from build123d import *

# Parameters (mm, degrees)
PAD_DEPTH   = 3.175
SKETCH001_R = 1.7
HOLE_DEPTH  = 3.176


with BuildPart() as part:
    # Sketch → Pad (new body)
    with BuildSketch(Plane.XY):
        with BuildLine():
            ThreePointArc((0, 3), (-3, 0), (0, -3))
            Line((0, -3), (35, -3))
            ThreePointArc((35, -3), (38, 0), (35, 3))
            Line((0, 3), (35, 3))
        make_face()
    extrude(amount=PAD_DEPTH)

    # Sketch001 (on Face6 of Pad) → Hole (cut, through all)
    with BuildSketch(Plane.XY.offset(3.175)):
        Circle(SKETCH001_R)
        with Locations((35, 0)):
            Circle(SKETCH001_R)
    extrude(amount=-HOLE_DEPTH, mode=Mode.SUBTRACT)


solid = part.part
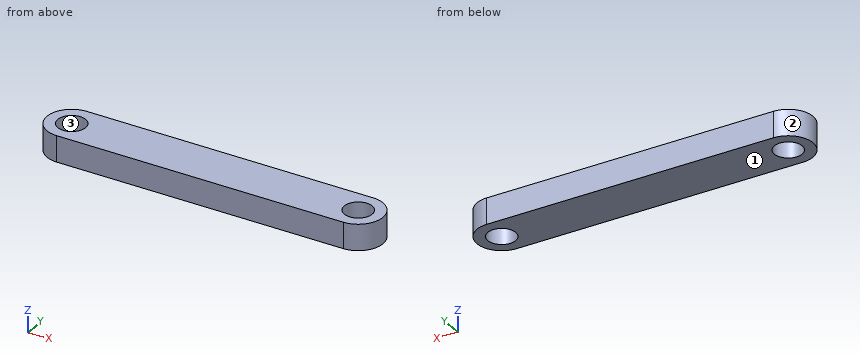
The listing builds one solid part. Answer for the finished solid, in the listing's coordinates (mm). Face numbers are marked on the shaded views. Coordinates: 2 decimals unless noted, no trailing zeros. Write each loop counter-clockwise with the first axis right and the second up, starting at its lowest first coordinate (ties: lowest second). Pieces come first, ordered by that corner, then holes. Notation, with made-up numbers: M 10.5,69.25 L 48.5,69.25 A25 cw 48.5,96.25 Z; hole C -12,-23 d1. An arc over 180 degrees is marked long. Write each question's results on one line, items separated by ' | '.
Item 1: For a pull along X with two mould halves and no side action, classify the marked faces 1, 2 and 3 as released by +X, released by -X, zero draft, split by the parting line, or undercut.
Answer below:
face 1: zero draft | face 2: released by -X | face 3: undercut
Item 2: The part is cut by section C-C on z = 2.55. Determine the outline of the cut face in (x, y).
Answer below:
outline: M 0,-3 L 35,-3 A3 ccw 35,3 L 0,3 A3 ccw Z; hole C 0,0 d3.4; hole C 35,0 d3.4
Item 3: Given P1, Ø1, axis at x = 13.5, y = -1.5, coming from the -Z side; P2, Ø2, axis at x = 0, y = 0, coming from the +Z side; P3, Ø1, axis at y = -1, z = 1, coming from the -X side, each flat-ended and moving along its own axis, determine where each tip first touches the part or whether it passes through.
Answer below:
P1: z = 0 | P2: through | P3: x = -2.96
Item 4: The part is cut by section B-B on x = 34.5. Determine the outline of the cut face in (y, z) (3 decimals), and give its area (3 significant figures).
Answer below:
outline: M -3,0 L -1.625,0 L -1.625,3.175 L -3,3.175 Z; M 1.625,0 L 3,0 L 3,3.175 L 1.625,3.175 Z | area: 8.73 mm2
Item 5: The part is cut by section A-A on y = 0. Determine the outline of the cut face in (x, z) (3 decimals).
Answer below:
outline: M -3,0 L -1.7,0 L -1.7,3.175 L -3,3.175 Z; M 1.7,0 L 33.3,0 L 33.3,3.175 L 1.7,3.175 Z; M 36.7,0 L 38,0 L 38,3.175 L 36.7,3.175 Z
Item 6: The part is cut by section D-D on y = 2.4. Determine the outline of the cut face in (x, z) (3 decimals).
Answer below:
outline: M -1.8,0 L 36.8,0 L 36.8,3.175 L -1.8,3.175 Z
Item 7: Consider probe 1 along X at (y, z) = (0.1, 2.25); probe 2 along X at (y, z) = (1.1, 2.65); probe 3 along Y at (x, z) = (35, 1.55). Determine where each line is inside the solid, lowest interval first. Write a range as [from, to].
Answer below:
probe 1: [-3, -1.7], [1.7, 33.3], [36.7, 38] | probe 2: [-2.79, -1.3], [1.3, 33.7], [36.3, 37.79] | probe 3: [-3, -1.7], [1.7, 3]
